Can you work these out from the model? Positions are in its coordinate system, mm. Give positions to 0.01 mm unless a question says otherwise; leave off trailing zeros. Loops run counter-clockwise (first coordinate to the right, second up) from the corner with the lowest first, then second, coordinate; pieces in that order, holes last. Notation, with made-up numbers: (-30, 42) - (14, 42) arc R17 cw to (14, 63) - close; hole circle Ø9 at (27, 37.5). An arc over 180 degrees is marked (long way). Answer as a JSON object with one key per item and string values. Group by question number.
Item 1: Suppose I cut it at A-A on x = 20. Write out the boundary of the cut face in (y, z), and give its area (3 significant figures).
Item 2: Suppose I cut it at B-B on z = 10.5. Write out the boundary of the cut face in (x, y) (3 decimals), and give its area (3 significant figures).
Item 3: Suppose I cut it at C-C on y = 3.75. Write out the boundary of the cut face in (x, z), and give its area (3 significant figures).
Item 4: Suppose I cut it at D-D on x = 4. Write out the boundary of the cut face in (y, z) (3 decimals).
Item 5: Please list where these lines run through material, in increasing order: L1, parallel to X at y = 5.25, z = 10.5; L2, parallel to X at y = 2.5, z = 12; L3, parallel to Y at x = 4, z = 9.75 (3 decimals).
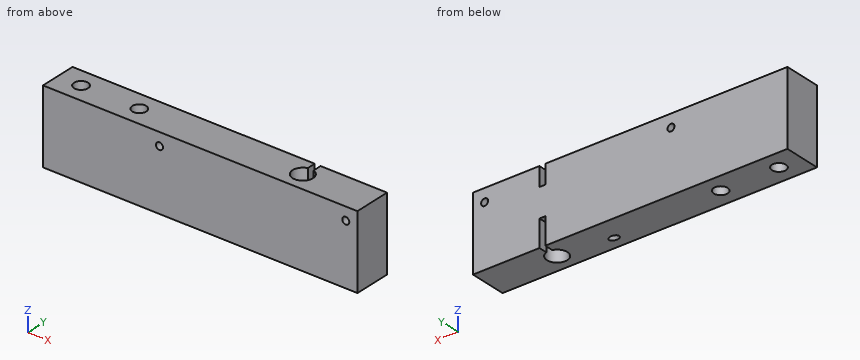
from build123d import *

# Parameters (mm, degrees)
SKETCH1_W           = 54
SKETCH1_H           = 6.35
BOSS_EXTRUDE1_DEPTH = 12.7
SKETCH3_W           = 1
SKETCH3_H           = 3.243111396
SKETCH3_H_2         = 4.577374163
CUT_EXTRUDE1_DEPTH  = 2
SKETCH4_R           = 1.75
CUT_EXTRUDE2_DEPTH  = 56.835584532
SKETCH5_R           = 0.6
CUT_EXTRUDE3_DEPTH  = 56.835584532
SKETCH6_R           = 1.2
CUT_EXTRUDE4_DEPTH  = 56.835584532
SKETCH12_R          = 0.6
CUT_EXTRUDE6_DEPTH  = 15


with BuildPart() as part:
    # Sketch1 → Boss-Extrude1 (new body)
    with BuildSketch(Plane.XY):
        with Locations((27, 3.175)):
            Rectangle(SKETCH1_W, SKETCH1_H)
    extrude(amount=BOSS_EXTRUDE1_DEPTH)

    # Sketch3 → Cut-Extrude1 (cut)
    with BuildSketch(Plane(origin=(0, 6.35, 0), x_dir=(1, 0, 0), z_dir=(0, 1, 0))):
        with Locations((42.087715046, -11.078444302)):
            Rectangle(SKETCH3_W, SKETCH3_H)
        with Locations((42.087715046, -2.288687081)):
            Rectangle(SKETCH3_W, SKETCH3_H_2)
    extrude(amount=-CUT_EXTRUDE1_DEPTH, mode=Mode.SUBTRACT)

    # Sketch4 → Cut-Extrude2 (cut, through all)
    with BuildSketch(Plane.XY.offset(12.7)):
        with Locations(Location((42.087715046, 3.175, 0), (0, 0, 73.398450401))):
            Circle(SKETCH4_R)
    extrude(amount=-CUT_EXTRUDE2_DEPTH, mode=Mode.SUBTRACT)

    # Sketch5 → Cut-Extrude3 (cut, through all)
    with BuildSketch(Plane(origin=(0, 6.35, 0), x_dir=(1, 0, 0), z_dir=(0, 1, 0))):
        with Locations(Location((52, -10.5, 0), (0, 0, 270))):
            Circle(SKETCH5_R)
        with Locations(Location((20, -10.5, 0), (0, 0, 270))):
            Circle(SKETCH5_R)
    extrude(amount=-CUT_EXTRUDE3_DEPTH, mode=Mode.SUBTRACT)

    # Sketch6 → Cut-Extrude4 (cut, through all)
    with BuildSketch(Plane.XY.offset(12.7)):
        with Locations((4, 3.175)):
            Circle(SKETCH6_R)
        with Locations((14, 3.175)):
            Circle(SKETCH6_R)
    extrude(amount=-CUT_EXTRUDE4_DEPTH, mode=Mode.SUBTRACT)

    # Sketch12 → Cut-Extrude6 (cut)
    with BuildSketch(Plane(origin=(25.944559134, 0, 23.885086629), x_dir=(-0.677303634830695, 0, 0.7357035994509805), z_dir=(-0.7357035994509805, 0, -0.677303634830695))):
        with Locations(Location((-22.399423471, 2.211286905, 0), (0, 0, 180))):
            Circle(SKETCH12_R)
    extrude(amount=CUT_EXTRUDE6_DEPTH, mode=Mode.SUBTRACT)


solid = part.part
Worked out:
{
 "1": {"outline": "(0, 0) - (6.35, 0) - (6.35, 9.9) - (0, 9.9) - close; (0, 11.1) - (6.35, 11.1) - (6.35, 12.7) - (0, 12.7) - close", "area": "73.0 mm2"},
 "2": {"outline": "(0, 0) - (19.4, 0) - (19.4, 6.35) - (0, 6.35) - close; (20.6, 0) - (51.4, 0) - (51.4, 6.35) - (42.588, 6.35) - (42.588, 4.852) arc R1.75 cw (long way) to (41.588, 4.852) - (41.588, 6.35) - (20.6, 6.35) - close; (52.6, 0) - (54, 0) - (54, 6.35) - (52.6, 6.35) - close; hole circle Ø2.4 at (4, 3.175); hole circle Ø2.4 at (14, 3.175)", "area": "308 mm2"},
 "3": {"outline": "(0, 0) - (2.95, 0) - (2.95, 12.7) - (0, 12.7) - close; (5.05, 0) - (12.95, 0) - (12.95, 12.7) - (5.05, 12.7) - close; (15.05, 0) - (40.43, 0) - (40.43, 12.7) - (15.05, 12.7) - close; (43.74, 0) - (54, 0) - (54, 12.7) - (43.74, 12.7) - close; hole circle Ø1.2 at (20, 10.5); hole circle Ø1.2 at (52, 10.5)", "area": "588 mm2"},
 "4": {"outline": "(0, 0) - (1.975, 0) - (1.975, 12.7) - (0, 12.7) - close; (4.375, 0) - (6.35, 0) - (6.35, 12.7) - (4.375, 12.7) - close"},
 "5": {"L1": "x = 0 to 19.4, 20.6 to 41.59, 42.59 to 51.4, 52.6 to 54", "L2": "x = 0 to 3.01, 4.99 to 13.01, 14.99 to 40.47, 43.7 to 54", "L3": "y = 0 to 1.975, 4.375 to 6.35"}
}
